Read the model definition and answer for the solid it produces. Units are mm, in the model's axes. A direction names the side the tool comes from. Coordinates: 2 decimals unless noted, no trailing zeros. Write each loop counter-clockwise with the first axis right and the second up, starting at its lowest first coordinate (ties: lowest second). Pieces come first, ordered by that corner, then holes. Notation, with made-up numbers: (-1.75, -15) -> (23.25, -15) arc R8 ccw to (23.25, -10) -> close; hole circle Ø1 at (30.25, -4). An arc over 180 degrees is marked (long way). Answer as a JSON object with one key per item and string values. Group by question number.
(1) Find section B-B (x = 56). Give the vertices of the cut face in (y, z).
(2) Which of the six approach directions +Z, -Z, +X, -X, +Y, -Y give full straight-line access (tool end or side, diameter ignored) to faces 1 (the face through (-56.552, -13, -60)), 2 (the face through (70.448, -13, -61)), 3 (the face through (8, -63, -21.091))?
(3) Flat-ended cylindrical pins translate along their axes: P1, Ø6, axis at x = 41, y = -150.5, coming from the -Z side; P2, Ø5.5, axis at x = 14.5, z = -22.5, coming from the -Y side; P3, Ø4, axis at y = -46.5, z = -24, coming from the +X side. Find the tip coordinate at first contact, or state that the pin passes through.
(4) For a pull along Z with two mould halves and no side action, classify faces 4 (the face through (6, -138, 38.132)), 5 (the face through (-65.94, -12.52, -45.5)), 6 (the face through (70.448, -89, 40)) as +Z half, -Z half, draft (parallel to the pull), parting line (faces both ways), or undercut.
(5) Find section A-A (y = -94). Give the vertices of the cut face in (x, z), then the cut area to 3 significant figures.
(6) Find section D-D (z = 32). Give the vertices of the cut face in (x, y).
(7) Straight lines are drawn through the part: L1, parallel to Z at x = -29.5, y = -87; L2, parallel to Y at x = 59.5, z = -53.5; L3, parallel to Z at x = -1.5, y = -163. For each, find the intervals that lie inside material, in ascending order.
(8) Find section C-C (y = -19.5). Give the vertices of the cut face in (x, z), then the cut area to 3 significant figures.
from build123d import *

# Parameters (mm, degrees)
F1_DEPTH  = 12.7
F0_W      = 63.5
F0_H      = 4.7856457531
F2_DEPTH  = 101.6
F3_DEPTH  = 254
F1_FACE_W = 127
F1_FACE_H = 46.801686123
F4_DEPTH  = 2.54
F6_DEPTH  = 25.4


# Not quite as in the source:
# - a feature of the source that left no trace in its solid (it failed there, or was rolled back) is left out


with BuildPart() as f1:
    # F0 (on Front) → F1 (new body)
    with BuildSketch(Plane.XZ):
        Polygon((6.9482082725, -25.8761684795), (-56.5517917275, -25.8761684795), (-56.5517917275, -47.4115650554), (-56.5517917275, -72.6778546025), (6.9482082725, -72.6778546025), align=None)
        Polygon((70.4482082725, -25.8761684795), (6.9482082725, -25.8761684795), (6.9482082725, -72.6778546025), (70.4482082725, -72.6778546025), (70.4482082725, -48.604208976), align=None)
    extrude(amount=F1_DEPTH)

    # F0 (on Front) → F2 (join)
    with BuildSketch(Plane.XZ):
        with Locations((-24.8017917275, -23.4833456029)):
            Rectangle(F0_W, F0_H)
        with Locations((38.6982082725, -23.4833456029)):
            Rectangle(F0_W, F0_H)
    extrude(amount=F2_DEPTH)

    # F0 (on Front) + F1_face (on face) → F4 (join)
    with BuildSketch(Plane.XZ):
        with BuildLine():
            Line((73.6600043416, 0), (70.4482082725, 0))
            Line((70.4482082725, 0), (70.4482082725, -21.0905227264))
            Line((70.4482082725, -21.0905227264), (70.4482082725, -25.8761684795))
            Line((70.4482082725, -25.8761684795), (70.4482082725, -48.604208976))
            Line((70.4482082725, -48.604208976), (73.6600043416, -48.604208976))
            ThreePointArc((73.6600043416, -48.604208976), (78.1501324021, -46.7443370366), (80.0100043416, -42.254208976))
            Line((80.0100043416, -42.254208976), (80.0100043416, -6.35))
            ThreePointArc((80.0100043416, -6.35), (78.1501324021, -1.8598719395), (73.6600043416, 0))
        make_face()
        with BuildLine():
            Line((-56.5517917275, -21.0905227264), (-56.5517917275, 0))
            Line((-56.5517917275, 0), (-61.3967882633, 0))
            ThreePointArc((-61.3967882633, 0), (-65.8869163239, -1.8598719395), (-67.7467882633, -6.35))
            Line((-67.7467882633, -6.35), (-67.7467882633, -41.0615650554))
            ThreePointArc((-67.7467882633, -41.0615650554), (-65.8869163239, -45.551693116), (-61.3967882633, -47.4115650554))
            Line((-61.3967882633, -47.4115650554), (-56.5517917275, -47.4115650554))
            Line((-56.5517917275, -47.4115650554), (-56.5517917275, -25.8761684795))
            Line((-56.5517917275, -25.8761684795), (-56.5517917275, -21.0905227264))
        make_face()
    with BuildSketch(Plane(origin=(6.9482082725, -12.7, -49.277011541), x_dir=(1, 0, 0), z_dir=(0, -1, 0))):
        Rectangle(F1_FACE_W, F1_FACE_H)
    extrude(amount=F4_DEPTH)



with BuildPart() as f3:
    # F0 (on Front) → F3 (new body)
    with BuildSketch(Plane.XZ):
        with BuildLine():
            ThreePointArc((-50.2017917275, 54.3221453975), (-54.6919197881, 52.462273458), (-56.5517917275, 47.9721453975))
            Line((-56.5517917275, 47.9721453975), (-56.5517917275, 38.1318327586))
            Line((-56.5517917275, 38.1318327586), (70.4482082725, 38.1318327586))
            Line((70.4482082725, 38.1318327586), (70.4482082725, 47.9721453975))
            ThreePointArc((70.4482082725, 47.9721453975), (68.588336333, 52.462273458), (64.0982082725, 54.3221453975))
            Line((64.0982082725, 54.3221453975), (-50.2017917275, 54.3221453975))
        make_face()
    extrude(amount=F3_DEPTH)


with BuildPart() as f1_1:
    add(f1.part)

    add(f3.part)  # F6 merges F3
    # F0 (on Front) → F6 (join)
    with BuildSketch(Plane.XZ):
        with BuildLine():
            ThreePointArc((-50.2017917275, 54.3221453975), (-54.6919197881, 52.462273458), (-56.5517917275, 47.9721453975))
            Line((-56.5517917275, 47.9721453975), (-56.5517917275, 38.1318327586))
            Line((-56.5517917275, 38.1318327586), (70.4482082725, 38.1318327586))
            Line((70.4482082725, 38.1318327586), (70.4482082725, 47.9721453975))
            ThreePointArc((70.4482082725, 47.9721453975), (68.588336333, 52.462273458), (64.0982082725, 54.3221453975))
            Line((64.0982082725, 54.3221453975), (-50.2017917275, 54.3221453975))
        make_face()
        Polygon((70.4482082725, 38.1318327586), (-56.5517917275, 38.1318327586), (-56.5517917275, 0), (-56.5517917275, -21.0905227264), (6.9482082725, -21.0905227264), (70.4482082725, -21.0905227264), (70.4482082725, 0), align=None)
        with BuildLine():
            Line((-56.5517917275, -21.0905227264), (-56.5517917275, 0))
            Line((-56.5517917275, 0), (-61.3967882633, 0))
            ThreePointArc((-61.3967882633, 0), (-65.8869163239, -1.8598719395), (-67.7467882633, -6.35))
            Line((-67.7467882633, -6.35), (-67.7467882633, -41.0615650554))
            ThreePointArc((-67.7467882633, -41.0615650554), (-65.8869163239, -45.551693116), (-61.3967882633, -47.4115650554))
            Line((-61.3967882633, -47.4115650554), (-56.5517917275, -47.4115650554))
            Line((-56.5517917275, -47.4115650554), (-56.5517917275, -25.8761684795))
            Line((-56.5517917275, -25.8761684795), (-56.5517917275, -21.0905227264))
        make_face()
        with BuildLine():
            Line((73.6600043416, 0), (70.4482082725, 0))
            Line((70.4482082725, 0), (70.4482082725, -21.0905227264))
            Line((70.4482082725, -21.0905227264), (70.4482082725, -25.8761684795))
            Line((70.4482082725, -25.8761684795), (70.4482082725, -48.604208976))
            Line((70.4482082725, -48.604208976), (73.6600043416, -48.604208976))
            ThreePointArc((73.6600043416, -48.604208976), (78.1501324021, -46.7443370366), (80.0100043416, -42.254208976))
            Line((80.0100043416, -42.254208976), (80.0100043416, -6.35))
            ThreePointArc((80.0100043416, -6.35), (78.1501324021, -1.8598719395), (73.6600043416, 0))
        make_face()
        Polygon((6.9482082725, -25.8761684795), (-56.5517917275, -25.8761684795), (-56.5517917275, -47.4115650554), (-56.5517917275, -72.6778546025), (6.9482082725, -72.6778546025), align=None)
        Polygon((70.4482082725, -25.8761684795), (6.9482082725, -25.8761684795), (6.9482082725, -72.6778546025), (70.4482082725, -72.6778546025), (70.4482082725, -48.604208976), align=None)
    extrude(amount=F6_DEPTH)


solid = f1_1.part
Results below:
{
 "1": {"outline": "(-254, 38.13) -> (-25.4, 38.13) -> (-25.4, -21.09) -> (-101.6, -21.09) -> (-101.6, -25.88) -> (-25.4, -25.88) -> (-25.4, -72.68) -> (0, -72.68) -> (0, 54.32) -> (-254, 54.32) -> close"},
 "2": {"face 1": "-Z, -X, +Y, -Y", "face 2": "-Z, +X, +Y, -Y", "face 3": "+X, -X, -Y"},
 "3": {"P1": "stops at z = 38.13", "P2": "stops at y = -101.6", "P3": "stops at x = 70.45"},
 "4": {"face 4": "undercut", "face 5": "-Z half", "face 6": "draft"},
 "5": {"outline": "(-56.55, -25.88) -> (70.45, -25.88) -> (70.45, -21.09) -> (-56.55, -21.09) -> close; (-56.55, 38.13) -> (70.45, 38.13) -> (70.45, 47.97) arc R6.35 ccw to (64.1, 54.32) -> (-50.2, 54.32) arc R6.35 ccw to (-56.55, 47.97) -> close", "area": "2,650 mm2"},
 "6": {"outline": "(-56.55, -25.4) -> (70.45, -25.4) -> (70.45, 0) -> (-56.55, 0) -> close"},
 "7": {"L1": "z = -25.88 to -21.09, 38.13 to 54.32", "L2": "y = -25.4 to 0", "L3": "z = 38.13 to 54.32"},
 "8": {"outline": "(-67.75, -41.06) arc R6.35 ccw to (-61.4, -47.41) -> (-56.55, -47.41) -> (-56.55, -72.68) -> (70.45, -72.68) -> (70.45, -48.6) -> (73.66, -48.6) arc R6.35 ccw to (80.01, -42.25) -> (80.01, -6.35) arc R6.35 ccw to (73.66, 0) -> (70.45, 0) -> (70.45, 47.97) arc R6.35 ccw to (64.1, 54.32) -> (-50.2, 54.32) arc R6.35 ccw to (-56.55, 47.97) -> (-56.55, 0) -> (-61.4, 0) arc R6.35 ccw to (-67.75, -6.35) -> close", "area": "17,100 mm2"}
}
